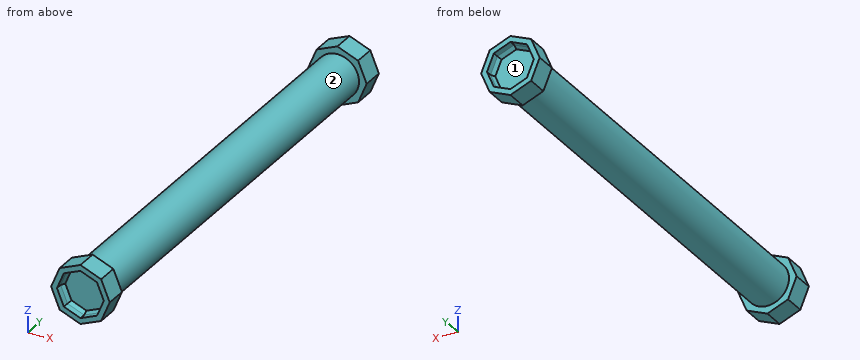
from build123d import *
from OCP.BRepFilletAPI import BRepFilletAPI_MakeChamfer

# Parameters (mm, degrees)
SKETCH1_R           = 12.7
BOSS_EXTRUDE1_DEPTH = 254
BOSS_EXTRUDE2_DEPTH = 12.7
BOSS_EXTRUDE3_DEPTH = 12.7
CUT_EXTRUDE1_DEPTH  = 6.35
CUT_EXTRUDE2_DEPTH  = 6.35
CHAMFER1_SIZE       = 2.54
CHAMFER1_SIZE2      = 1.184421452
CHAMFER2_SIZE       = 2.54
CHAMFER2_SIZE2      = 1.184421452


with BuildPart() as part:
    # Sketch1 → Boss-Extrude1 (new body)
    with BuildSketch(Plane(origin=(0, 0, 0), x_dir=(1, 0, 0), z_dir=(0, 1, 0))):
        with Locations(Location((0, 0, 0), (0, 0, 270))):
            Circle(SKETCH1_R)
    extrude(amount=BOSS_EXTRUDE1_DEPTH)

    # Sketch2 → Boss-Extrude2 (add)
    with BuildSketch(Plane(origin=(0, 254, 0), x_dir=(1, 0, 0), z_dir=(0, 1, 0))):
        Polygon((0, 17.18297618), (-12.150198978, 12.150198978), (-17.18297618, 0), (-12.150198978, -12.150198978), (0, -17.18297618), (12.150198978, -12.150198978), (17.18297618, 0), (12.150198978, 12.150198978), align=None)
    extrude(amount=BOSS_EXTRUDE2_DEPTH)

    # Sketch3 → Boss-Extrude3 (add)
    with BuildSketch(Plane.XZ):
        Polygon((0, 17.18297618), (-12.150198978, 12.150198978), (-17.18297618, 0), (-12.150198978, -12.150198978), (0, -17.18297618), (12.150198978, -12.150198978), (17.18297618, 0), (12.150198978, 12.150198978), align=None)
    extrude(amount=BOSS_EXTRUDE3_DEPTH)

    # Sketch4 → Cut-Extrude1 (cut)
    with BuildSketch(Plane(origin=(0, 266.7, 0), x_dir=(1, 0, 0), z_dir=(0, 1, 0))):
        Polygon((0, 13.746380944), (-9.720159182, 9.720159182), (-13.746380944, 0), (-9.720159182, -9.720159182), (0, -13.746380944), (9.720159182, -9.720159182), (13.746380944, 0), (9.720159182, 9.720159182), align=None)
    extrude(amount=-CUT_EXTRUDE1_DEPTH, mode=Mode.SUBTRACT)

    # Sketch5 → Cut-Extrude2 (cut)
    with BuildSketch(Plane.XZ.offset(12.7)):
        Polygon((0, 13.746380944), (-9.720159182, 9.720159182), (-13.746380944, 0), (-9.720159182, -9.720159182), (0, -13.746380944), (9.720159182, -9.720159182), (13.746380944, 0), (9.720159182, 9.720159182), align=None)
    extrude(amount=-CUT_EXTRUDE2_DEPTH, mode=Mode.SUBTRACT)

    # Chamfer1: one chamfer whose edges measure the first distance from different faces: ONE call of the kernel's chamfer builder (chamfer() names one face for all edges)
    chamfer1_edges_1 = [part.edges().sort_by_distance(p)[0] for p in [
        (4.860079591, -6.35, 11.733270063),
    ]]
    chamfer1_side_1 = [part.faces().sort_by_distance(p)[0] for p in [
        (4.860079591, -9.525, 11.733270063),
    ]]
    chamfer1_edges_2 = [part.edges().sort_by_distance(p)[0] for p in [
        (11.733270063, -6.35, 4.860079591),
    ]]
    chamfer1_side_2 = [part.faces().sort_by_distance(p)[0] for p in [
        (11.733270063, -9.525, 4.860079591),
    ]]
    chamfer1_edges_3 = [part.edges().sort_by_distance(p)[0] for p in [
        (11.733270063, -6.35, -4.860079591),
    ]]
    chamfer1_side_3 = [part.faces().sort_by_distance(p)[0] for p in [
        (11.733270063, -9.525, -4.860079591),
    ]]
    chamfer1_edges_4 = [part.edges().sort_by_distance(p)[0] for p in [
        (4.860079591, -6.35, -11.733270063),
    ]]
    chamfer1_side_4 = [part.faces().sort_by_distance(p)[0] for p in [
        (4.860079591, -9.525, -11.733270063),
    ]]
    chamfer1_edges_5 = [part.edges().sort_by_distance(p)[0] for p in [
        (-4.860079591, -6.35, -11.733270063),
    ]]
    chamfer1_side_5 = [part.faces().sort_by_distance(p)[0] for p in [
        (-4.860079591, -9.525, -11.733270063),
    ]]
    chamfer1_edges_6 = [part.edges().sort_by_distance(p)[0] for p in [
        (-11.733270063, -6.35, -4.860079591),
    ]]
    chamfer1_side_6 = [part.faces().sort_by_distance(p)[0] for p in [
        (-11.733270063, -9.525, -4.860079591),
    ]]
    chamfer1_edges_7 = [part.edges().sort_by_distance(p)[0] for p in [
        (-11.733270063, -6.35, 4.860079591),
    ]]
    chamfer1_side_7 = [part.faces().sort_by_distance(p)[0] for p in [
        (-11.733270063, -9.525, 4.860079591),
    ]]
    chamfer1_edges_8 = [part.edges().sort_by_distance(p)[0] for p in [
        (-4.860079591, -6.35, 11.733270063),
    ]]
    chamfer1_side_8 = [part.faces().sort_by_distance(p)[0] for p in [
        (-4.860079591, -9.525, 11.733270063),
    ]]
    chamfer1 = BRepFilletAPI_MakeChamfer(part.part.solid().wrapped)
    for e in chamfer1_edges_1:
        chamfer1.Add(CHAMFER1_SIZE, CHAMFER1_SIZE2, e.wrapped, chamfer1_side_1[0].wrapped)  # the first distance lies on this face
    for e in chamfer1_edges_2:
        chamfer1.Add(CHAMFER1_SIZE, CHAMFER1_SIZE2, e.wrapped, chamfer1_side_2[0].wrapped)  # the first distance lies on this face
    for e in chamfer1_edges_3:
        chamfer1.Add(CHAMFER1_SIZE, CHAMFER1_SIZE2, e.wrapped, chamfer1_side_3[0].wrapped)  # the first distance lies on this face
    for e in chamfer1_edges_4:
        chamfer1.Add(CHAMFER1_SIZE, CHAMFER1_SIZE2, e.wrapped, chamfer1_side_4[0].wrapped)  # the first distance lies on this face
    for e in chamfer1_edges_5:
        chamfer1.Add(CHAMFER1_SIZE, CHAMFER1_SIZE2, e.wrapped, chamfer1_side_5[0].wrapped)  # the first distance lies on this face
    for e in chamfer1_edges_6:
        chamfer1.Add(CHAMFER1_SIZE, CHAMFER1_SIZE2, e.wrapped, chamfer1_side_6[0].wrapped)  # the first distance lies on this face
    for e in chamfer1_edges_7:
        chamfer1.Add(CHAMFER1_SIZE, CHAMFER1_SIZE2, e.wrapped, chamfer1_side_7[0].wrapped)  # the first distance lies on this face
    for e in chamfer1_edges_8:
        chamfer1.Add(CHAMFER1_SIZE, CHAMFER1_SIZE2, e.wrapped, chamfer1_side_8[0].wrapped)  # the first distance lies on this face
    add(Compound.cast(chamfer1.Shape()), mode=Mode.REPLACE)

    # Chamfer2: one chamfer whose edges measure the first distance from different faces: ONE call of the kernel's chamfer builder (chamfer() names one face for all edges)
    chamfer2_edges_1 = [part.edges().sort_by_distance(p)[0] for p in [
        (4.860079591, 260.35, -11.733270063),
    ]]
    chamfer2_side_1 = [part.faces().sort_by_distance(p)[0] for p in [
        (4.860079591, 263.525, -11.733270063),
    ]]
    chamfer2_edges_2 = [part.edges().sort_by_distance(p)[0] for p in [
        (11.733270063, 260.35, -4.860079591),
    ]]
    chamfer2_side_2 = [part.faces().sort_by_distance(p)[0] for p in [
        (11.733270063, 263.525, -4.860079591),
    ]]
    chamfer2_edges_3 = [part.edges().sort_by_distance(p)[0] for p in [
        (11.733270063, 260.35, 4.860079591),
    ]]
    chamfer2_side_3 = [part.faces().sort_by_distance(p)[0] for p in [
        (11.733270063, 263.525, 4.860079591),
    ]]
    chamfer2_edges_4 = [part.edges().sort_by_distance(p)[0] for p in [
        (4.860079591, 260.35, 11.733270063),
    ]]
    chamfer2_side_4 = [part.faces().sort_by_distance(p)[0] for p in [
        (4.860079591, 263.525, 11.733270063),
    ]]
    chamfer2_edges_5 = [part.edges().sort_by_distance(p)[0] for p in [
        (-4.860079591, 260.35, 11.733270063),
    ]]
    chamfer2_side_5 = [part.faces().sort_by_distance(p)[0] for p in [
        (-4.860079591, 263.525, 11.733270063),
    ]]
    chamfer2_edges_6 = [part.edges().sort_by_distance(p)[0] for p in [
        (-11.733270063, 260.35, 4.860079591),
    ]]
    chamfer2_side_6 = [part.faces().sort_by_distance(p)[0] for p in [
        (-11.733270063, 263.525, 4.860079591),
    ]]
    chamfer2_edges_7 = [part.edges().sort_by_distance(p)[0] for p in [
        (-11.733270063, 260.35, -4.860079591),
    ]]
    chamfer2_side_7 = [part.faces().sort_by_distance(p)[0] for p in [
        (-11.733270063, 263.525, -4.860079591),
    ]]
    chamfer2_edges_8 = [part.edges().sort_by_distance(p)[0] for p in [
        (-4.860079591, 260.35, -11.733270063),
    ]]
    chamfer2_side_8 = [part.faces().sort_by_distance(p)[0] for p in [
        (-4.860079591, 263.525, -11.733270063),
    ]]
    chamfer2 = BRepFilletAPI_MakeChamfer(part.part.solid().wrapped)
    for e in chamfer2_edges_1:
        chamfer2.Add(CHAMFER2_SIZE, CHAMFER2_SIZE2, e.wrapped, chamfer2_side_1[0].wrapped)  # the first distance lies on this face
    for e in chamfer2_edges_2:
        chamfer2.Add(CHAMFER2_SIZE, CHAMFER2_SIZE2, e.wrapped, chamfer2_side_2[0].wrapped)  # the first distance lies on this face
    for e in chamfer2_edges_3:
        chamfer2.Add(CHAMFER2_SIZE, CHAMFER2_SIZE2, e.wrapped, chamfer2_side_3[0].wrapped)  # the first distance lies on this face
    for e in chamfer2_edges_4:
        chamfer2.Add(CHAMFER2_SIZE, CHAMFER2_SIZE2, e.wrapped, chamfer2_side_4[0].wrapped)  # the first distance lies on this face
    for e in chamfer2_edges_5:
        chamfer2.Add(CHAMFER2_SIZE, CHAMFER2_SIZE2, e.wrapped, chamfer2_side_5[0].wrapped)  # the first distance lies on this face
    for e in chamfer2_edges_6:
        chamfer2.Add(CHAMFER2_SIZE, CHAMFER2_SIZE2, e.wrapped, chamfer2_side_6[0].wrapped)  # the first distance lies on this face
    for e in chamfer2_edges_7:
        chamfer2.Add(CHAMFER2_SIZE, CHAMFER2_SIZE2, e.wrapped, chamfer2_side_7[0].wrapped)  # the first distance lies on this face
    for e in chamfer2_edges_8:
        chamfer2.Add(CHAMFER2_SIZE, CHAMFER2_SIZE2, e.wrapped, chamfer2_side_8[0].wrapped)  # the first distance lies on this face
    add(Compound.cast(chamfer2.Shape()), mode=Mode.REPLACE)


solid = part.part
Could you check a few things on this model? Use its own coordinates, in mm. Face numbers are marked on the shaded views. Give positions to 0.01 mm unless a question says otherwise; leave off trailing zeros. Order: outer loops, then holes, each group sorted by start corner. A loop starts at its lowest first (then second) coordinate and runs counter-clockwise, first axis right, second up.
Item 1: If we mould it in two halves opening along Z, with no side actions, what happens to the marked faces 1 and 2? For each: pulls with the +Z half, pulls with the -Z half, needs draft (parallel to the pull), parting line crosses it, or undercut.
Item 2: If we section it at B-B, the plane y = 79: Write out the boundary of the cut face in (x, z), plus the area to 3 significant figures.
Item 3: If we section it at A-A, the plane z = -6: Write out the boundary of the cut face in (x, y), plus the area to 3 significant figures.
Item 4: I'm going to push flat-ended pins straight in: pin 1 (10 mm diameter, centred on x = 13, y = 219.5, fed in from -Z); pin 2 (12.5 mm diameter, centred on x = -2.5, z = -2.5, fed in from -Y); pin 3 (10 mm diameter, centred on x = -1, z = 3.5, fed in from +Y). Where does each tip first touch, or does it pass through?
Item 5: If we section it at C-C, the plane x = 6.5: Write out the boundary of the cut face in (y, z).
Item 6: I need wall thicknesses on line 1 (Y direction, x = 13, z = -4); line 2 (Z direction, x = -1, y = 134); line 3 (Y direction, x = 11, z = 0.5). Which ranges of each line are inside material? Lowest first, please.
Values:
1. face 1: undercut
1. face 2: parting line crosses it
2. outline: circle Ø25.4 at (0, 0)
2. area: 507 mm2
3. outline: (-14.7, -12.7) - (-11.26, -12.7) - (-11.26, -8.89) - (-9.98, -6.35) - (9.98, -6.35) - (11.26, -8.89) - (11.26, -12.7) - (14.7, -12.7) - (14.7, 0) - (11.19, 0) - (11.19, 254) - (14.7, 254) - (14.7, 266.7) - (11.26, 266.7) - (11.26, 262.89) - (9.98, 260.35) - (-9.98, 260.35) - (-11.26, 262.89) - (-11.26, 266.7) - (-14.7, 266.7) - (-14.7, 254) - (-11.19, 254) - (-11.19, 0) - (-14.7, 0) - close
3. area: 6,150 mm2
4. pin 1: stops at z = -9.86
4. pin 2: stops at y = -6.35
4. pin 3: stops at y = 260.35
5. outline: (-12.7, -14.49) - (0, -14.49) - (0, -10.91) - (254, -10.91) - (254, -14.49) - (266.7, -14.49) - (266.7, -11.05) - (262.89, -11.05) - (260.35, -9.77) - (260.35, 9.77) - (262.89, 11.05) - (266.7, 11.05) - (266.7, 14.49) - (254, 14.49) - (254, 10.91) - (0, 10.91) - (0, 14.49) - (-12.7, 14.49) - (-12.7, 11.05) - (-8.89, 11.05) - (-6.35, 9.77) - (-6.35, -9.77) - (-8.89, -11.05) - (-12.7, -11.05) - close
6. line 1: y = -12.7 to 0, 254 to 266.7
6. line 2: z = -12.66 to 12.66
6. line 3: y = -6.35 to 260.35
